Geometry check sheet. Reference: the model listing, model coordinates, mm. A direction names the side the tool comes from. Round coordinates to 2 decimals unless told otherwise and drop trailing zeros. Loops run counter-clockwise (first coordinate to the right, second up) from the corner with the lowest first, then second, coordinate; pieces in that order, holes last. Notation, with made-up numbers: (24, 70.25) -> (30, 70.25) arc R21 cw to (30, 92.25) -> close; hole circle Ø1 at (-18.75, 32). An arc over 180 degrees is marked (long way). Use one line per item in the form item = value.
from build123d import *

# Parameters (mm, degrees)
BOSS_EXTRUDE1_DEPTH = 10


with BuildPart() as part:
    # Sketch1 → Revolve1 (revolve)
    with BuildSketch(Plane.XY, mode=Mode.PRIVATE) as revolve1_sk:
        Polygon((0, 0), (-28, 0), (-28, 14), (-26, 14), (-26, 9), (-23, 9), (-23, 14), (-21, 14), (-21, 4), (0, 4), align=None)
    revolve(revolve1_sk.sketch.rotate(Axis((0, 4, 0), (0, -1, 0)), 270), axis=Axis((0, 4, 0), (0, -1, 0)))

    # Sketch3 → Boss-Extrude1 (add)
    with BuildSketch(Plane(origin=(0, 4, 0), x_dir=(1, 0, 0), z_dir=(0, 1, 0))):
        with BuildLine():
            ThreePointArc((-3.829930462, -3.214285714), (-4.516748393, -2.687346066), (-5.361902647, -2.5))
            Line((-5.361902647, -2.5), (-6.280127387, -2.5))
            ThreePointArc((-6.280127387, -2.5), (-7.637061373, -1.969261773), (-8.273818621, -0.658730159))
            ThreePointArc((-8.273818621, -0.658730159), (-8.3, 0), (-8.273818621, 0.658730159))
            ThreePointArc((-8.273818621, 0.658730159), (-7.637061373, 1.969261773), (-6.280127387, 2.5))
            Line((-6.280127387, 2.5), (-5.361902647, 2.5))
            ThreePointArc((-5.361902647, 2.5), (-4.516748393, 2.687346066), (-3.829930462, 3.214285714))
            ThreePointArc((-3.829930462, 3.214285714), (-3.686233368, 3.378118346), (-3.535533906, 3.535533906))
            ThreePointArc((-3.535533906, 3.535533906), (-3.378118346, 3.686233368), (-3.214285714, 3.829930462))
            ThreePointArc((-3.214285714, 3.829930462), (-2.687346066, 4.516748393), (-2.5, 5.361902647))
            Line((-2.5, 5.361902647), (-2.5, 6.280127387))
            ThreePointArc((-2.5, 6.280127387), (-1.969261773, 7.637061373), (-0.658730159, 8.273818621))
            ThreePointArc((-0.658730159, 8.273818621), (0, 8.3), (0.658730159, 8.273818621))
            ThreePointArc((0.658730159, 8.273818621), (1.969261773, 7.637061373), (2.5, 6.280127387))
            Line((2.5, 6.280127387), (2.5, 5.361902647))
            ThreePointArc((2.5, 5.361902647), (2.687346066, 4.516748393), (3.214285714, 3.829930462))
            ThreePointArc((3.214285714, 3.829930462), (3.378118346, 3.686233368), (3.535533906, 3.535533906))
            ThreePointArc((3.535533906, 3.535533906), (3.686233368, 3.378118346), (3.829930462, 3.214285714))
            ThreePointArc((3.829930462, 3.214285714), (4.516748393, 2.687346066), (5.361902647, 2.5))
            Line((5.361902647, 2.5), (6.280127387, 2.5))
            ThreePointArc((6.280127387, 2.5), (7.637061373, 1.969261773), (8.273818621, 0.658730159))
            ThreePointArc((8.273818621, 0.658730159), (8.3, 0), (8.273818621, -0.658730159))
            ThreePointArc((8.273818621, -0.658730159), (7.637061373, -1.969261773), (6.280127387, -2.5))
            Line((6.280127387, -2.5), (5.361902647, -2.5))
            ThreePointArc((5.361902647, -2.5), (4.516748393, -2.687346066), (3.829930462, -3.214285714))
            ThreePointArc((3.829930462, -3.214285714), (3.686233368, -3.378118346), (3.535533906, -3.535533906))
            ThreePointArc((3.535533906, -3.535533906), (3.378118346, -3.686233368), (3.214285714, -3.829930462))
            ThreePointArc((3.214285714, -3.829930462), (2.687346066, -4.516748393), (2.5, -5.361902647))
            Line((2.5, -5.361902647), (2.5, -6.280127387))
            ThreePointArc((2.5, -6.280127387), (1.969261773, -7.637061373), (0.658730159, -8.273818621))
            ThreePointArc((0.658730159, -8.273818621), (0, -8.3), (-0.658730159, -8.273818621))
            ThreePointArc((-0.658730159, -8.273818621), (-1.969261773, -7.637061373), (-2.5, -6.280127387))
            Line((-2.5, -6.280127387), (-2.5, -5.361902647))
            ThreePointArc((-2.5, -5.361902647), (-2.687346066, -4.516748393), (-3.214285714, -3.829930462))
            ThreePointArc((-3.214285714, -3.829930462), (-3.378118346, -3.686233368), (-3.535533906, -3.535533906))
            ThreePointArc((-3.535533906, -3.535533906), (-3.686233368, -3.378118346), (-3.829930462, -3.214285714))
        make_face()
    extrude(amount=BOSS_EXTRUDE1_DEPTH)


solid = part.part
1. Tool access check on faces 1 (the cylindrical face through (2.68, 8.93, -4.53)), 2 (the flat face through (0, 14, 0)). Record the directions out of +Z, -Z, +X, -X, +Y, -Y that give a thin tool (end or side, any length) a straight path to the whole face; none if there is none.
Return value:
face_1 = +Y
face_2 = +Z, -Z, +X, -X, +Y
2. Section check B-B (x = 0). Record the boundary of the cut face in (y, z).
Return value:
outline = (0, -28) -> (14, -28) -> (14, -26) -> (9, -26) -> (9, -23) -> (14, -23) -> (14, -21) -> (4, -21) -> (4, -8.3) -> (14, -8.3) -> (14, 8.3) -> (4, 8.3) -> (4, 21) -> (14, 21) -> (14, 23) -> (9, 23) -> (9, 26) -> (14, 26) -> (14, 28) -> (0, 28) -> close
3. Material ranges on line 1 along X through (y, z) = (9.5, 0); line 2 along Z through (x, y) = (11.5, 9.5); line 3 along X through (y, z) = (9.75, -17.5), recorded low to high.
Return value:
line_1 = -28 to -26, -23 to -21, -8.3 to 8.3, 21 to 23, 26 to 28
line_2 = -25.53 to -23.32, -19.92 to -17.57, 17.57 to 19.92, 23.32 to 25.53
line_3 = -21.86 to -19.23, -14.92 to -11.61, 11.61 to 14.92, 19.23 to 21.86
4. Section check A-A (y = 12.5). Count the separate pieces of the cut face and the enclosed holes in it, then the cut area to 3 significant figures.
Return value:
separate_pieces = 3
enclosed_holes = 2
area = 759 mm2
5. Gauge pin test, flat ends, axial feed: pin 1 (1 mm diameter, centred on y = 8.5, z = -6, fed in from +X); pin 2 (1 mm diameter, centred on y = 8.5, z = -6, fed in from -X); pin 3 (0.7 mm diameter, centred on x = 6, y = 7, fed in from -Z). Record the tip position at first contact, or that the pin passes through.
Return value:
pin_1 = 27.45
pin_2 = -27.45
pin_3 = -27.42
6. Section check C-C (z = 0). Record the boundary of the cut face in (x, y), then the cut area to 3 significant figures.
Return value:
outline = (-28, 0) -> (28, 0) -> (28, 14) -> (26, 14) -> (26, 9) -> (23, 9) -> (23, 14) -> (21, 14) -> (21, 4) -> (8.3, 4) -> (8.3, 14) -> (-8.3, 14) -> (-8.3, 4) -> (-21, 4) -> (-21, 14) -> (-23, 14) -> (-23, 9) -> (-26, 9) -> (-26, 14) -> (-28, 14) -> close
area = 500 mm2
7. Mould release check, pull along Z, two halves, no side actions. Record for faces 3 (the cylindrical face through (27.334, 7.098, -6.07)), 4 (the cylindrical face through (-2.69, 8.93, -4.51)), 5 (the flat face through (0, 0, 0)): released by +Z, released by -Z, zero draft, split by the parting line, or undercut.
Return value:
face_3 = split by the parting line
face_4 = undercut
face_5 = zero draft
